```python
from build123d import *

# Parameters (mm, degrees)
SKETCH1_W                = 8.5
SKETCH1_H                = 8.5
BOSS_EXTRUDE1_DEPTH      = 3
CUT_EXTRUDE1_DEPTH       = 3
SHELL2_T                 = 0.5
SKETCH3_R                = 1
CUT_EXTRUDE2_DEPTH       = 0.5
BOSS_EXTRUDE2_DEPTH      = 0.15
SKETCH5_R                = 1
CUT_EXTRUDE3_DEPTH       = 0.01
BOSS_EXTRUDE3_DEPTH      = 0.01
BOSS_EXTRUDE3_DEPTH_BACK = 0.1
SKETCH6_W                = 1
SKETCH6_H                = 1
SKETCH7_R                = 0.25
CUT_EXTRUDE4_DEPTH       = 0.1


with BuildPart() as part:
    # Sketch1 → Boss-Extrude1 (new body)
    with BuildSketch(Plane(origin=(0, 0, 0), x_dir=(1, 0, 0), z_dir=(0, 1, 0))):
        Rectangle(SKETCH1_W, SKETCH1_H)
    extrude(amount=BOSS_EXTRUDE1_DEPTH)

    # Sketch2 → Cut-Extrude1 (cut)
    with BuildSketch(Plane(origin=(0, 3, 0), x_dir=(1, 0, 0), z_dir=(0, 1, 0))):
        Polygon((-4.25, 2.75), (-2.75, 4.25), (-4.25, 4.25), align=None)
        Polygon((4.25, 4.25), (4.25, 2.75), (2.75, 4.25), align=None)
        Polygon((4.25, -2.75), (2.75, -4.25), (4.25, -4.25), align=None)
        Polygon((-4.25, -4.25), (-4.25, -2.75), (-2.75, -4.25), align=None)
    extrude(amount=-CUT_EXTRUDE1_DEPTH, mode=Mode.SUBTRACT)

    # Shell2 (no face opened: a closed hollow body)
    add(offset(amount=-SHELL2_T, mode=Mode.PRIVATE), mode=Mode.SUBTRACT)

    # Sketch3 → Cut-Extrude2 (cut)
    with BuildSketch(Plane(origin=(0, 3, 0), x_dir=(1, 0, 0), z_dir=(0, 1, 0))):
        with Locations(Location((0, 0, 0), (0, 0, 270))):
            Circle(SKETCH3_R)
    extrude(amount=-CUT_EXTRUDE2_DEPTH, mode=Mode.SUBTRACT)

    # Sketch4 → Boss-Extrude2 (add)
    with BuildSketch(Plane.XZ):
        Polygon((3.48749395, 2.426833778), (4.030330086, 2.969669914), (2.969669914, 4.030330086), (2.426833778, 3.48749395), align=None)
        with BuildLine():
            Line((4.030330086, 2.969669914), (4.053179375, 2.992519203))
            Line((4.053179375, 2.992519203), (4.194600731, 3.13394056))
            Line((4.194600731, 3.13394056), (4.194600731, 3.994600731))
            ThreePointArc((4.194600731, 3.994600731), (4.136022088, 4.136022088), (3.994600731, 4.194600731))
            Line((3.994600731, 4.194600731), (3.13394056, 4.194600731))
            Line((3.13394056, 4.194600731), (2.969669914, 4.030330086))
            Line((2.969669914, 4.030330086), (4.030330086, 2.969669914))
        make_face()
        Polygon((4.194600731, -3.13394056), (4.053179375, -2.992519203), (4.030330086, -2.969669914), (2.969669914, -4.030330086), (3.13394056, -4.194600731), align=None)
        Polygon((2.969669914, -4.030330086), (4.030330086, -2.969669914), (3.48749395, -2.426833778), (2.426833778, -3.48749395), align=None)
        with BuildLine():
            Line((-4.030330086, -2.969669914), (-4.053179375, -2.992519203))
            Line((-4.053179375, -2.992519203), (-4.194600731, -3.13394056))
            Line((-4.194600731, -3.13394056), (-4.194600731, -3.994600731))
            ThreePointArc((-4.194600731, -3.994600731), (-4.136022088, -4.136022088), (-3.994600731, -4.194600731))
            Line((-3.994600731, -4.194600731), (-3.13394056, -4.194600731))
            Line((-3.13394056, -4.194600731), (-2.969669914, -4.030330086))
            Line((-2.969669914, -4.030330086), (-4.030330086, -2.969669914))
        make_face()
        Polygon((-3.48749395, -2.426833778), (-4.030330086, -2.969669914), (-2.969669914, -4.030330086), (-2.426833778, -3.48749395), align=None)
        Polygon((-2.969669914, 4.030330086), (-4.030330086, 2.969669914), (-3.48749395, 2.426833778), (-2.426833778, 3.48749395), align=None)
        with BuildLine():
            Line((-4.194600731, 3.13394056), (-4.053179375, 2.992519203))
            Line((-4.053179375, 2.992519203), (-4.030330086, 2.969669914))
            Line((-4.030330086, 2.969669914), (-2.969669914, 4.030330086))
            Line((-2.969669914, 4.030330086), (-3.13394056, 4.194600731))
            Line((-3.13394056, 4.194600731), (-3.994600731, 4.194600731))
            ThreePointArc((-3.994600731, 4.194600731), (-4.136022088, 4.136022088), (-4.194600731, 3.994600731))
            Line((-4.194600731, 3.994600731), (-4.194600731, 3.13394056))
        make_face()
    extrude(amount=BOSS_EXTRUDE2_DEPTH)

    # Sketch5 → Cut-Extrude3 (cut)
    with BuildSketch(Plane(origin=(0, 3, 0), x_dir=(1, 0, 0), z_dir=(0, 1, 0))):
        with Locations(Location((-2.25, 2.25, 0), (0, 0, 270))):
            Circle(SKETCH5_R)
        with BuildLine():
            ThreePointArc((-3, 2.3), (-2.970710678, 2.370710678), (-2.9, 2.4))
            Line((-2.9, 2.4), (-2.4, 2.4))
            Line((-2.4, 2.4), (-2.4, 2.9))
            ThreePointArc((-2.4, 2.9), (-2.370710678, 2.970710678), (-2.3, 3))
            Line((-2.3, 3), (-2.2, 3))
            ThreePointArc((-2.2, 3), (-2.129289322, 2.970710678), (-2.1, 2.9))
            Line((-2.1, 2.9), (-2.1, 2.4))
            Line((-2.1, 2.4), (-1.6, 2.4))
            ThreePointArc((-1.6, 2.4), (-1.529289322, 2.370710678), (-1.5, 2.3))
            Line((-1.5, 2.3), (-1.5, 2.2))
            ThreePointArc((-1.5, 2.2), (-1.529289322, 2.129289322), (-1.6, 2.1))
            Line((-1.6, 2.1), (-2.1, 2.1))
            Line((-2.1, 2.1), (-2.1, 1.6))
            ThreePointArc((-2.1, 1.6), (-2.129289322, 1.529289322), (-2.2, 1.5))
            Line((-2.2, 1.5), (-2.3, 1.5))
            ThreePointArc((-2.3, 1.5), (-2.370710678, 1.529289322), (-2.4, 1.6))
            Line((-2.4, 1.6), (-2.4, 2.1))
            Line((-2.4, 2.1), (-2.9, 2.1))
            ThreePointArc((-2.9, 2.1), (-2.970710678, 2.129289322), (-3, 2.2))
            Line((-3, 2.2), (-3, 2.3))
        make_face(mode=Mode.SUBTRACT)
    extrude(amount=-CUT_EXTRUDE3_DEPTH, mode=Mode.SUBTRACT)

    # Sketch6 → Boss-Extrude3 (add, two sides: drawn at the far end of the back side and taken through both)
    with BuildSketch(Plane.XZ.offset(-BOSS_EXTRUDE3_DEPTH_BACK)):
        with Locations((3.8, 0.9)):
            Rectangle(SKETCH6_W, SKETCH6_H)
        with Locations((3.8, -0.9)):
            Rectangle(SKETCH6_W, SKETCH6_H)
    extrude(amount=BOSS_EXTRUDE3_DEPTH + BOSS_EXTRUDE3_DEPTH_BACK)

    # Sketch7 → Cut-Extrude4 (cut)
    with BuildSketch(Plane.XZ):
        with Locations(Location((0, 2.8, 0), (0, 0, 270))):
            Circle(SKETCH7_R)
        with Locations(Location((0, -2.8, 0), (0, 0, 90))):
            Circle(SKETCH7_R)
    extrude(amount=-CUT_EXTRUDE4_DEPTH, mode=Mode.SUBTRACT)


solid = part.part
```
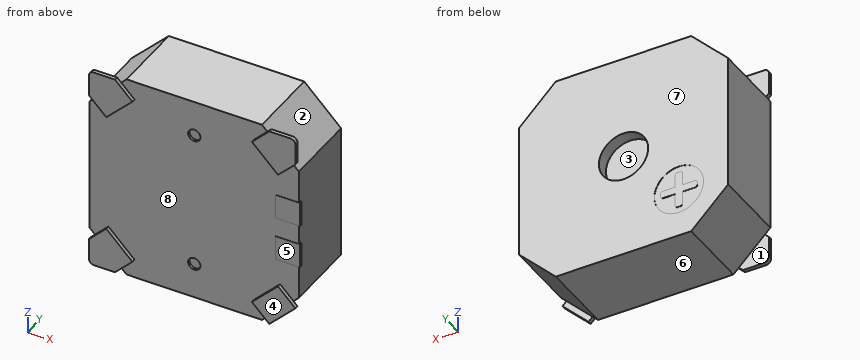
Geometry check sheet. Reference: the model listing, model coordinates, mm. Face numbers are marked on the shaded views. A direction names the side the tool comes from. Coordinates: 2 decimals unless noted, no trailing zeros. Order: outer loops, then holes, each group sorted by start corner. A loop starts at its lowest first (then second) coordinate and runs counter-clockwise, first axis right, second up. Notation, with made-up numbers: (2, -29) - (49, -29) arc R10 ccw to (49, -15) - close; hole circle Ø9 at (82, 66). An arc over 180 degrees is marked (long way). Answer as a JSON object with one key per item and string values. Group by question number.
Item 1: Scan lines: probe 1 along Y at (x, z) = (-3.5, 1.75); probe 2 along Z at (x, y) = (2.5, 1.2). Record each from-to range of solid material in increasing order.
Item 2: Draft check along Z on the marked faces 6, 7 and 8. Enter one of: +Z half, -Z half, draft (parallel to the pull), parting line (faces both ways), or undercut.
Item 3: Sectioned sample at B-B, the plane x = 2. Record the cut outline in (y, z).
Item 4: Sectioned sample at A-A, the plane y = 2.6. Record the cut outline in (x, z).
Item 5: Tool access check on the marked faces 1, 2, 3, 4 and 5. Record the directions out of +Z, -Z, +X, -X, +Y, -Y that give a thin tool (end or side, any length) a straight path to the whole face; none if there is none.
Item 6: Depth check by flat-ended pin: pin 1 Ø5 at (x, z) = (-2.5, -1.5) entering from +Y; pin 2 Ø2.5 at (x, z) = (-0.5, 0) entering from -Y. Enter the tip coordinate at first touch or a pass-through.
Item 7: Sectioned sample at C-C, the plane z = 0. Record the cut outline in (x, y).
Resolved:
{
 "1": {"probe 1": "0 to 0.5, 2.5 to 3", "probe 2": "-4.25 to -3.75, 3.75 to 4.25"},
 "2": {"face 6": "-Z half", "face 7": "draft", "face 8": "undercut"},
 "3": {"outline": "(0, -4.25) - (3, -4.25) - (3, 4.25) - (0, 4.25) - close; hole (0.5, -3.75) - (2.5, -3.75) - (2.5, 3.75) - (0.5, 3.75) - close"},
 "4": {"outline": "(-4.25, -2.75) - (-2.75, -4.25) - (2.75, -4.25) - (4.25, -2.75) - (4.25, 2.75) - (2.75, 4.25) - (-2.75, 4.25) - (-4.25, 2.75) - close; hole circle Ø2 at (0, 0)"},
 "5": {"face 1": "-Z, -X, +Y", "face 2": "+Z, +X, +Y", "face 3": "none", "face 4": "+Z, -Z, +X, -X, -Y", "face 5": "+X, -X, -Y"},
 "6": {"pin 1": "y = 3", "pin 2": "y = 0"},
 "7": {"outline": "(-4.25, 0) - (4.25, 0) - (4.25, 3) - (1, 3) - (1, 2.5) - (3.75, 2.5) - (3.75, 0.5) - (-3.75, 0.5) - (-3.75, 2.5) - (-1, 2.5) - (-1, 3) - (-4.25, 3) - close"}
}
